```python
from build123d import *

# Parameters (mm, degrees)
BOSS_EXTRUDE1_DEPTH = 12.7
FILLET1_R           = 1.5875


with BuildPart() as part:
    # Sketch3 → Boss-Extrude1 (new, symmetric)
    with BuildSketch(Plane.XY):
        Polygon((3.175, 19.05), (0, 19.05), (0, 0), (19.05, 0), (19.05, 3.175), (3.175, 3.175), align=None)
    extrude(amount=BOSS_EXTRUDE1_DEPTH, both=True)

    # Fillet1
    fillet1_edges = [part.edges().sort_by_distance(p)[0] for p in [
        (3.175, 3.175, 0),
        (19.05, 3.175, 0),
        (3.175, 19.05, 0),
    ]]
    fillet(fillet1_edges, radius=FILLET1_R)


solid = part.part
```
The listing builds one solid part. Answer for the finished solid, in the listing's coordinates (mm). A direction names the side the tool comes from. Coordinates: 2 decimals unless noted, no trailing zeros. Loops run counter-clockwise (first coordinate to the right, second up) from the corner with the lowest first, then second, coordinate; pieces in that order, holes last. Notation, with made-up numbers: (72, 6.5) - (115, 6.5) arc R10 cw to (115, 20.5) - close; hole circle Ø11 at (72.25, 35.5). An arc over 180 degrees is marked (long way). Write item = value, one per line.
1) Each of these flat-tipped pins is pushed along its axis until it touches: P1, Ø10, axis at x = 12.5, z = 4.5, coming from the +Y side (3 decimals); P2, Ø4, axis at y = 2.5, z = 5.5, coming from the -X side; P3, Ø6.5, axis at y = 9.5, z = -2, coming from the +X side (3 decimals). Where does it stop, or does it pass through?
Responses:
P1 = 3.175
P2 = 0
P3 = 3.175
2) Which of the six approach directions +Z, -Z, +X, -X, +Y, -Y give full straight-line access (tool end or side, diameter ignored) to faces 1 (the face through (19.05, 1, 0)), 2 (the face through (11, 3.175, 0))?
Responses:
face_1 = +Z, -Z, +X, +Y, -Y
face_2 = +Z, -Z, +X, +Y
3) Find the intervals of material crossed by line 1 along X through (y, z) = (7.25, -5.25) (3 decimals); line 2 along X through (y, z) = (4, -9.75), in increasing order.
Responses:
line_1 = 0 to 3.175
line_2 = 0 to 3.37
4) Section B-B (x = 5.75) is taken. Determine the outline of the cut face in (y, z) (3 decimals), plus the area to 3 significant figures.
Responses:
outline = (0, -12.7) - (3.175, -12.7) - (3.175, 12.7) - (0, 12.7) - close
area = 80.6 mm^2
